CAD build for the part. Positions are in the model's coordinates, mm. A direction names the side the tool comes from. Coordinates: 2 decimals unless noted, no trailing zeros. Loops run counter-clockwise (first coordinate to the right, second up) from the corner with the lowest first, then second, coordinate; pieces in that order, holes last. Notation, with made-up numbers: (8, 15.5) - (28, 15.5) arc R8 ccw to (28, 19.5) - close; hole circle Ø10 at (83.5, 46). An arc over 180 degrees is marked (long way). Put each result on its own line as item: value.
```python
from build123d import *

# Parameters (mm, degrees)
SKETCH_1_W          = 42
SKETCH_1_H          = 42
EXTRUDE_1_DEPTH     = 40
SKETCH_3_R          = 1.5
CUT_EXTRUDE_1_DEPTH = 50.819674828
SKETCH_4_R          = 11
EXTRUDE_2_DEPTH     = 2
SKETCH_5_R          = 2.5
EXTRUDE_3_DEPTH     = 24


with BuildPart() as part:
    # 스케치1 → 보스-돌출1 (new body)
    with BuildSketch(Plane(origin=(0, 0, 0), x_dir=(1, 0, 0), z_dir=(0, 1, 0))):
        Rectangle(SKETCH_1_W, SKETCH_1_H)
    extrude(amount=EXTRUDE_1_DEPTH)

    # 스케치3 → 컷-돌출1 (cut, through all)
    with BuildSketch(Plane(origin=(0, 40, 0), x_dir=(1, 0, 0), z_dir=(0, 1, 0))):
        with Locations(Location((-15.5, 15.5, 0), (0, 0, 270))):
            Circle(SKETCH_3_R)
        with Locations(Location((15.5, 15.5, 0), (0, 0, 270))):
            Circle(SKETCH_3_R)
        with Locations(Location((15.5, -15.5, 0), (0, 0, 270))):
            Circle(SKETCH_3_R)
        with Locations(Location((-15.5, -15.5, 0), (0, 0, 270))):
            Circle(SKETCH_3_R)
    extrude(amount=-CUT_EXTRUDE_1_DEPTH, mode=Mode.SUBTRACT)

    # 스케치4 → 보스-돌출2 (add)
    with BuildSketch(Plane(origin=(0, 40, 0), x_dir=(1, 0, 0), z_dir=(0, 1, 0))):
        with Locations(Location((0, 0, 0), (0, 0, 90))):
            Circle(SKETCH_4_R)
    extrude(amount=EXTRUDE_2_DEPTH)

    # 스케치5 → 보스-돌출3 (add)
    with BuildSketch(Plane(origin=(0, 42, 0), x_dir=(1, 0, 0), z_dir=(0, 1, 0))):
        with Locations(Location((0, 0, 0), (0, 0, 270))):
            Circle(SKETCH_5_R)
    extrude(amount=EXTRUDE_3_DEPTH)


solid = part.part
```
Q1. Wall check: L1, parallel to X at y = 11, z = -15.5; L2, parallel to Z at x = 15, y = 11; L3, parallel to Y at x = -14, z = 3.5. Give the ranges that are in metal, low to high. Write a range as from..to.
Determined:
L1: -21..-17, -14..14, 17..21
L2: -21..-16.91, -14.09..14.09, 16.91..21
L3: 0..40
Q2. Mould opens along Z. For faces 3 (the cylindrical face through (10.74, 40.99, 2.38)), 4 (the flat face through (21, 20, 0)), 5 (the cylindrical face through (15.57, 20.28, 14)) say: +Z half, -Z half, draft (parallel to the pull), parting line (faces both ways), or undercut.
Determined:
face 3: parting line
face 4: draft
face 5: undercut
Q3. Pin check, flat tips, straight feed: pin 1 Ø1.8 at (x, z) = (-15.5, 15.5) entering from -Y; pin 2 Ø4 at (x, z) = (-15.5, -15.5) entering from +Y; pin 3 Ø8 at (x, z) = (-5, -16.5) entering from -Y. Stop position of each tip, or through.
Determined:
pin 1: through
pin 2: y = 40
pin 3: y = 0
Q4. Tool access for faces 1 (the flat face through (0, 20, -21)), 2 (the cylindrical face through (-2.44, 53.83, -0.54)): list every direction of +Z, -Z, +X, -X, +Y, -Y with a clear straight run to the whole face (end or side of a thin tool).
Determined:
face 1: -Z, +X, -X, +Y, -Y
face 2: +Y
Q5. Slice it at B-B, the plane y = 21.5. Give the cut face in (x, z).
Determined:
outline: (-21, -21) - (21, -21) - (21, 21) - (-21, 21) - close; hole circle Ø3 at (-15.5, -15.5); hole circle Ø3 at (-15.5, 15.5); hole circle Ø3 at (15.5, -15.5); hole circle Ø3 at (15.5, 15.5)
Q6. Slice it at A-A, the plane z = 15.5. Give the cut face in (x, y), then the cut area to 3 significant figures.
Determined:
outline: (-21, 0) - (-17, 0) - (-17, 40) - (-21, 40) - close; (-14, 0) - (14, 0) - (14, 40) - (-14, 40) - close; (17, 0) - (21, 0) - (21, 40) - (17, 40) - close
area: 1,440 mm2
Q7. Slice it at C-C, the plane x = 15.5. Give the cut face in (y, z).
Determined:
outline: (0, -21) - (40, -21) - (40, -17) - (0, -17) - close; (0, -14) - (40, -14) - (40, 14) - (0, 14) - close; (0, 17) - (40, 17) - (40, 21) - (0, 21) - close
Q8. Slice it at D-D, the plane x = 0. Give the cut face in (y, z).
Determined:
outline: (0, -21) - (40, -21) - (40, -11) - (42, -11) - (42, -2.5) - (66, -2.5) - (66, 2.5) - (42, 2.5) - (42, 11) - (40, 11) - (40, 21) - (0, 21) - close
